from build123d import *

# Parameters (mm, degrees)
CROQUIS1_W              = 190
CROQUIS1_H              = 250
SALIENTE_EXTRUIR1_DEPTH = 5
REDONDEO1_R             = 10
CROQUIS2_W              = 150
CROQUIS2_H              = 230
SALIENTE_EXTRUIR2_DEPTH = 10


with BuildPart() as part:
    # Croquis1 → Saliente-Extruir1 (new body)
    with BuildSketch(Plane(origin=(0, 0, 0), x_dir=(1, 0, 0), z_dir=(0, 1, 0))):
        with Locations((95, 125)):
            Rectangle(CROQUIS1_W, CROQUIS1_H)
    extrude(amount=SALIENTE_EXTRUIR1_DEPTH)

    # Redondeo1
    redondeo1_edges = [part.edges().sort_by_distance(p)[0] for p in [
        (0, 2.5, -250),
        (190, 2.5, -250),
        (190, 2.5, 0),
        (0, 2.5, 0),
    ]]
    fillet(redondeo1_edges, radius=REDONDEO1_R)

    # Croquis2 → Saliente-Extruir2 (add)
    with BuildSketch(Plane.XZ):
        with Locations((95, -125)):
            Rectangle(CROQUIS2_W, CROQUIS2_H)
    extrude(amount=SALIENTE_EXTRUIR2_DEPTH)


solid = part.part
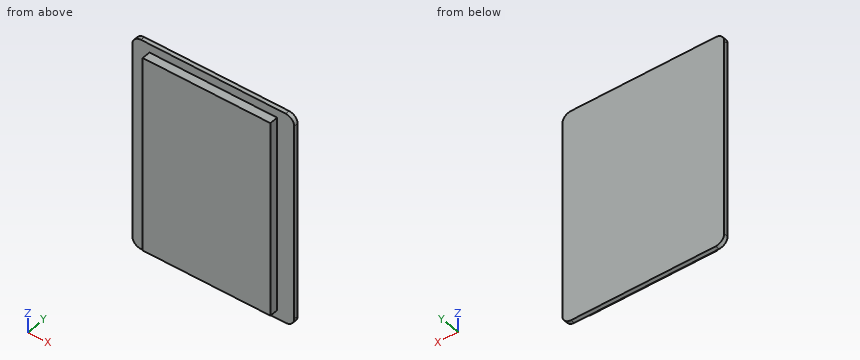
The model under review builds one solid part; all positions refer to its coordinate system, in mm. Give positions to 0.01 mm unless a question says otherwise; leave off trailing zeros. Order: outer loops, then holes, each group sorted by start corner. A loop starts at its lowest first (then second) coordinate and runs counter-clockwise, first axis right, second up. Notation, with made-up numbers: (77.25, 64.25) -> (118.25, 64.25) arc R32 ccw to (118.25, 96.25) -> close; hole circle Ø3 at (-40, 45.5). An arc over 180 degrees is marked (long way). Write item = value, one per line. Start each with the question number.
(1) For L1, parallel to Z at x = 59.5, y = -2.75; L2, parallel to X at y = -5.5, z = -121; L3, parallel to Y at x = 178, z = -189, list the stretches that pass through material, from the lowest coordinate up. Write a range as from..to.
(2) Take a section at A-A (z = -184.5). Write out the cut boundary in (x, y), plus the area to 3 significant figures.
(3) Take a section at C-C (y = -6.25). Write out the cut boundary in (x, z), plus the area to 3 significant figures.
(4) Take a section at B-B (x = 156.5). Write out the cut boundary in (y, z), plus the area to 3 significant figures.
(5) For pin 1 Ø1.5 at (y, z) = (-3, -222) entering from +X; pin 2 Ø1.5 at (x, y) = (115, -5) entering from -Z; pin 3 Ø3 at (y, z) = (-6.5, -92) entering from -X, all flat-tipped, find the tip position at first contact; note any pin that passes through.
Returned:
q1.L1 = -240..-10
q1.L2 = 20..170
q1.L3 = 0..5
q2.outline = (0, 0) -> (20, 0) -> (20, -10) -> (170, -10) -> (170, 0) -> (190, 0) -> (190, 5) -> (0, 5) -> close
q2.area = 2,450 mm²
q3.outline = (20, -240) -> (170, -240) -> (170, -10) -> (20, -10) -> close
q3.area = 34,500 mm²
q4.outline = (-10, -240) -> (0, -240) -> (0, -250) -> (5, -250) -> (5, 0) -> (0, 0) -> (0, -10) -> (-10, -10) -> close
q4.area = 3,550 mm²
q5.pin_1 = 170
q5.pin_2 = -240
q5.pin_3 = 20
